Input: part model. Units: mm. Frame: model coordinates. Round coordinates to 2 decimals unless told otherwise and drop trailing zeros. One line per item, written item: value. Start each with the question number.
Autodesk Inventor part; units mm, degrees
ref_plane "YZ Plane" through (0, 0, 0) normal (1, 0, 0) x (0, 1, 0)
ref_plane "XZ Plane" through (0, 0, 0) normal (0, 1, 0) x (-1, 0, 0)
ref_plane "XY Plane" through (0, 0, 0) normal (0, 0, 1) x (1, 0, 0)
sketch "Sketch1" plane through (0, 0, 0) normal (0, 0, 1) x (1, 0, 0)
  line L0 (-60, 42.5) -> (60, 42.5)
  line L1 (60, 42.5) -> (60, -42.5)
  line L2 (60, -42.5) -> (-60, -42.5)
  line L3 (-60, -42.5) -> (-60, 42.5)
  point P0 (0, 0)
  point P1 (0, 42.5)
  point P2 (60, 0)
  dimension "d0" = 120
  dimension "d1" = 85
extrude "Extrusion1" add sketch "Sketch1" along normal blind 5
sketch "Sketch2" plane through (0, 0, 5) normal (0, 0, 1) x (1, 0, 0)
  line L0 (-55, 37.5) -> (55, 37.5) construction
  line L1 (55, 37.5) -> (55, -37.5) construction
  line L2 (55, -37.5) -> (-55, -37.5) construction
  line L3 (-55, -37.5) -> (-55, 37.5) construction
  point P0 (0, 0)
  point P1 (0, 37.5)
  point P2 (55, 0)
  point P3 (-21.4621, 82.9295)
  dimension "d4" = 110
  dimension "d5" = 75
hole "Hole1" at (-55, 37.5, 5) at (55, 37.5, 5) at (55, -37.5, 5) at (-55, -37.5, 5) at (-21.4621, 82.9295, 5) direction (0, 0, -1) diameter 3 end through all
fillet "Fillet1" radius 4 4 edges at (60, 42.5, 2.5) (60, -42.5, 2.5) (-60, 42.5, 2.5) (-60, -42.5, 2.5)
properties part number "duo-esp32-pcb-outline"
Item 1: Line query: L1, parallel to X at y = 37.5, z = 3.2; L2, parallel to Y at x = -55, z = 2.2. Output: solid intervals per line, ascending.
Item 2: First-contact query: pin 1 Ø2.5 at (x, y) = (-55, -37.5) entering from -Z. Flat tip, straight axial feed; report the tip coordinate or a pass-through.
Item 3: Pull-direction query (Y, two-part tool) for faces 1 (the face through (-54.1, -36.3, 2.5)), 2 (the face through (58.797, -41.359, 2.535)), 3 (the face through (-1, 1, 5)); classes: released by +Y, released by -Y, zero draft, split by the parting line, or undercut.
Geometry results:
1. L1: x = -60 to -56.5, -53.5 to 53.5, 56.5 to 60
1. L2: y = -42.5 to -39, -36 to 36, 39 to 42.5
2. pin 1: passes through
3. face 1: undercut
3. face 2: released by -Y
3. face 3: zero draft
